The listing builds one solid part. Answer for the finished solid, in the listing's coordinates (mm). Coordinates: 2 decimals unless noted, no trailing zeros. Order: outer loops, then holes, each group sorted by start corner. A loop starts at its lowest first (then second) coordinate and runs counter-clockwise, first axis right, second up. Notation, with made-up numbers: (69.25, 67.25) -> (107.25, 67.25) arc R6 ccw to (107.25, 71.25) -> close; hole circle Ø6 at (85, 65). An arc over 180 degrees is marked (long way). Return JSON: item names as keys, results as strings.
from build123d import *

# Parameters (mm, degrees)
BOSS_EXTRUDE1_DEPTH      = 23
F_8_0_8_DIAMETER_HOLE1_D = 8
FILLET1_R                = 3.99999999


with BuildPart() as part:
    # Sketch1 → Boss-Extrude1 (new body)
    with BuildSketch(Plane.XZ.offset(7.5)):
        with BuildLine():
            Line((6.9, 0), (-6.9, 0))
            ThreePointArc((-6.9, 0), (-4.163490138, -4.720459639), (-3e-09, -8.247012535))
            ThreePointArc((-3e-09, -8.247012535), (4.163490136, -4.720459641), (6.9, 0))
        make_face()
    extrude(amount=-BOSS_EXTRUDE1_DEPTH)

    # Ø8.0 (8) Diameter Hole1 (through all)
    with Locations(Plane.XY):
        with Locations((0, 0)):
            Hole(F_8_0_8_DIAMETER_HOLE1_D / 2)

    # Fillet1
    fillet1_edges = [part.edges().sort_by_distance(p)[0] for p in [
        (-3e-09, 9.75, -8.247012535),
        (-3e-09, -5.75, -8.247012535),
    ]]
    fillet(fillet1_edges, radius=FILLET1_R)


solid = part.part
1. The part is cut by section C-C on z = -4. Give the vertices of the cut face in (x, y), and give its area (3 significant figures).
Answer block:
{"outline": "(-4.73, -7.5) -> (4.73, -7.5) -> (4.73, 15.5) -> (-4.73, 15.5) -> close; hole circle Ø8 at (0, 0)", "area": "167 mm2"}
2. Determine the mould class of faces 1 (the face through (4, 0, -3)), 2 (the face through (0, -7.5, -3)), 3 (the face through (0, 15.5, -3)), 4 (the face through (2, 4, 0)) for opening direction Y: pulls with the +Y half, pulls with the -Y half, needs draft (parallel to the pull), parting line crosses it, or undercut.
Answer block:
{"face 1": "undercut", "face 2": "pulls with the -Y half", "face 3": "pulls with the +Y half", "face 4": "needs draft"}
3. Consider line 1 (Y direction, x = 0, z = -5.5); line 2 (Y direction, x = 1.75, z = -0.25); line 3 (X direction, y = 0, z = -3). Determine where each line is inside the solid, lowest interval first. Write a range as from..to.
Answer block:
{"line 1": "y = -7.5..-4, 4..15.5", "line 2": "y = -7.5..-3.6, 3.6..15.5", "line 3": "x = -5.42..-4, 4..5.42"}
4. Each of these flat-tipped pins is pushed along its axis until it touches: pin 1 Ø2 at (y, z) = (10, -4) entering from +X; pin 2 Ø3 at (y, z) = (1, -4) entering from +X. Where does it stop, or does it pass through?
Answer block:
{"pin 1": "stops at x = 5.42", "pin 2": "stops at x = 5.72"}
5. The part is cut by section D-D on x = -3. Give the vertices of the cut face in (y, z), and give its area (3 significant figures).
Answer block:
{"outline": "(-7.5, -5.97) -> (-2.65, -5.97) -> (-2.65, 0) -> (-7.5, 0) -> close; (2.65, -5.97) -> (15.5, -5.97) -> (15.5, 0) -> (2.65, 0) -> close", "area": "106 mm2"}
6. The part is cut by section B-B on y = -1. Give the vertices of the cut face in (x, z).
Answer block:
{"outline": "(-6.9, 0) arc R16 ccw to (-3.87, -5.06) -> (-3.87, 0) -> close; (3.87, -5.06) arc R16 ccw to (6.9, 0) -> (3.87, 0) -> close"}
7. The part is cut by section A-A on x = 3.75. Give the vertices of the cut face in (y, z), and give its area (3 significant figures).
Answer block:
{"outline": "(-7.5, -5.2) -> (-1.39, -5.2) -> (-1.39, 0) -> (-7.5, 0) -> close; (1.39, -5.2) -> (15.5, -5.2) -> (15.5, 0) -> (1.39, 0) -> close", "area": "105 mm2"}
